```python
from build123d import *

# Parameters (mm, degrees)
BOSS_EXTRU_1_DEPTH = 0.8
BOSS_EXTRU_2_DEPTH = 20


with BuildPart() as part:
    # Esquisse1 → Boss.-Extru.1 (new body)
    with BuildSketch(Plane.XY):
        Polygon((22.85, 64.904088569), (-22.85, 64.904088569), (-34.25, 56.354088569), (-22.85, 47.804088569), (22.85, 47.804088569), (34.25, 56.354088569), align=None)
    extrude(amount=BOSS_EXTRU_1_DEPTH)

    # Esquisse2 → Boss.-Extru.2 (add)
    with BuildSketch(Plane.XY.offset(0.8)):
        Polygon((34.25, 56.354088569), (22.85, 64.904088569), (-22.85, 64.904088569), (-34.25, 56.354088569), (-22.85, 47.804088569), (22.85, 47.804088569), align=None)
        Polygon((-22.583333333, 64.104088569), (-32.916666667, 56.354088569), (-22.583333333, 48.604088569), (22.583333333, 48.604088569), (32.916666667, 56.354088569), (22.583333333, 64.104088569), align=None, mode=Mode.SUBTRACT)
    extrude(amount=BOSS_EXTRU_2_DEPTH)


solid = part.part
```
CAD build for the part. Positions are in the model's coordinates, mm. A direction names the side the tool comes from. Coordinates: 2 decimals unless noted, no trailing zeros. Write each loop counter-clockwise with the first axis right and the second up, starting at its lowest first coordinate (ties: lowest second). Pieces come first, ordered by that corner, then holes. Notation, with made-up numbers: (-36, -25.75) -> (-13, -25.75) arc R32 ccw to (-13, 3.25) -> close; hole circle Ø3 at (50.25, 25.25). An arc over 180 degrees is marked (long way). Return JSON: item names as keys, results as strings. Group by question number.
Q1. Cut at B-B, the plane z = 10.75. Give the cut face in (x, y), then the cut area to 3 significant figures.
Q2. Flat gauge pins, fed straight in: pin 1 (3 mm diameter, centred on x = 15, y = 51, fed in from +Z); pin 2 (5 mm diameter, centred on x = -9.5, y = 62, fed in from -Z); pin 3 (1 mm diameter, centred on y = 62.5, z = 3.5, fed in from +X). Where does each tip first touch, or does it go through?
Q3. Cut at A-A, the plane x = -19.5. Give the cut face in (y, z), then the cut area to 3 significant figures.
Q4. Cut at C-C, the plane y = 54. Give the cut face in (x, z), then the cut area to 3 significant figures.
Q5. Drill centre lines: line 1 (Y direction, x = 15, z = 17.5); line 2 (Z direction, x = -8, y = 59); line 3 (X direction, y = 62.5, z = 9). Where is each one in solid material? Low to high.
Q6. Which spindle directions (+Z, -Z, +X, -X, +Y, -Y) get a long thin tool onto all of the face, cutting with end or side? Do faces 5 (the face through (-27.68, 60.28, 10.66)), 6 (the face through (0, 47.804, 10)). Say none if no direction does.
Q7. Pull direction Y, two halves, no side cores. Call faces 1 (the face through (28.47, 52.02, 10.25)), 2 (the face through (-5, 48, 20.8)), 3 (the face through (-28.47, 60.69, 10.25)), 4 (the face through (0, 48.604, 11)): released by +Y, released by -Y, zero draft, split by the parting line, or undercut.
Returned:
{
 "1": {"outline": "(-34.25, 56.35) -> (-22.85, 47.8) -> (22.85, 47.8) -> (34.25, 56.35) -> (22.85, 64.9) -> (-22.85, 64.9) -> close; hole (-32.92, 56.35) -> (-22.58, 48.6) -> (22.58, 48.6) -> (32.92, 56.35) -> (22.58, 64.1) -> (-22.58, 64.1) -> close", "area": "116 mm2"},
 "2": {"pin 1": "stops at z = 0.8", "pin 2": "stops at z = 0", "pin 3": "stops at x = 26.72"},
 "3": {"outline": "(47.8, 0) -> (64.9, 0) -> (64.9, 20.8) -> (64.1, 20.8) -> (64.1, 0.8) -> (48.6, 0.8) -> (48.6, 20.8) -> (47.8, 20.8) -> close", "area": "45.7 mm2"},
 "4": {"outline": "(-31.11, 0) -> (31.11, 0) -> (31.11, 20.8) -> (29.78, 20.8) -> (29.78, 0.8) -> (-29.78, 0.8) -> (-29.78, 20.8) -> (-31.11, 20.8) -> close", "area": "103 mm2"},
 "5": {"line 1": "y = 47.8 to 48.6, 64.1 to 64.9", "line 2": "z = 0 to 0.8", "line 3": "x = -26.06 to -24.72, 24.72 to 26.06"},
 "6": {"face 5": "+Z", "face 6": "+Z, -Z, +X, -X, -Y"},
 "7": {"face 1": "released by -Y", "face 2": "zero draft", "face 3": "released by +Y", "face 4": "undercut"}
}
